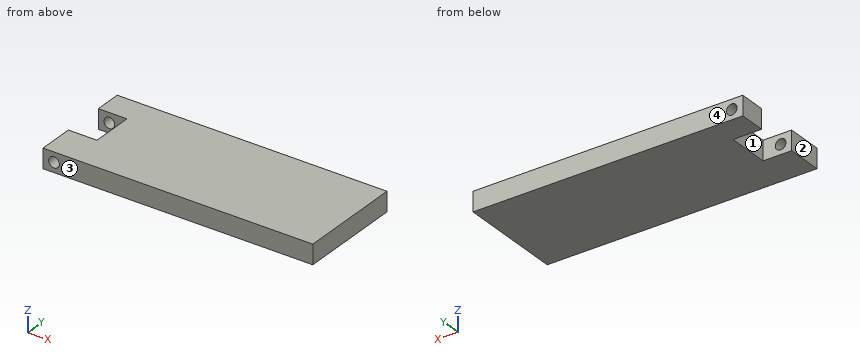
from build123d import *

# Parameters (mm, degrees)
F0_W     = 87.707184
F0_H     = 34.12497
F1_DEPTH = 6.35
F2_W     = 9.312924
F2_H     = 13.797991
F3_DEPTH = 6.35
F4_R     = 1.73945
F5_DEPTH = 34.12497


with BuildPart() as f1:
    # F0 (on Top) → F1 (new body)
    with BuildSketch(Plane.XY):
        with Locations((43.853592, 17.062485)):
            Rectangle(F0_W, F0_H)
    extrude(amount=F1_DEPTH)

    # F2 (on face) → F3 (cut, through all)
    with BuildSketch(Plane.XY.offset(6.35)):
        with Locations((4.656462, 18.549588)):
            Rectangle(F2_W, F2_H)
    extrude(amount=-F3_DEPTH, mode=Mode.SUBTRACT)

    # F4 (on face) → F5 (cut, through all)
    with BuildSketch(Plane(origin=(0, 34.12497, 0), x_dir=(-1, 0, 0), z_dir=(0, 1, 0))):
        with Locations((-3.584127, 3.175)):
            Circle(F4_R)
    extrude(amount=-F5_DEPTH, mode=Mode.SUBTRACT)


solid = f1.part
Work out the finished part from the listing and answer in its coordinate system (mm). Face numbers are marked on the shaded views. Coordinates: 2 decimals unless noted, no trailing zeros. Write each loop counter-clockwise with the first axis right and the second up, starting at its lowest first coordinate (ties: lowest second). Pieces come first, ordered by that corner, then holes. Notation, with made-up numbers: M 49,69.5 L 69,69.5 A20 ccw 69,92.5 Z; hole C 33,40.25 d4. An arc over 180 degrees is marked long. Answer as CSV lines item,"result". Start each with the question number.
Item 1: Determine the mould class of the marked faces 1, 2, 3 and 4 for opening direction Y: released by +Y, released by -Y, zero draft, split by the parting line, or undercut.
Item 2: Consider L1, parallel to X at y = 26.5, z = 3; L2, parallel to X at y = 14, z = 5; L3, parallel to X at y = 5, z = 4.25. Determine where each line is inside the solid, lowest interval first.
Item 3: Flat-ended cylindrical pins translate along their axes: P1, Ø1, axis at y = 23.5, z = 1, coming from the -X side; P2, Ø1.9, axis at x = 4.5, z = 2.5, coming from the +Y side. Find the tip coordinate at first contact, or state that the pin passes through.
Item 4: Section A-A on y = 31.5 is taken. Write down the section's boundary in (x, z) (3 decimals).
Item 5: Section B-B on y = 24.5 is taken. Write down the section's boundary in (x, z), and give its area (3 significant figures).
Checks:
1,face 1,"undercut"
1,face 2,"zero draft"
1,face 3,"released by -Y"
1,face 4,"released by +Y"
2,L1,"x = 0 to 1.85, 5.31 to 87.71"
2,L2,"x = 9.31 to 87.71"
2,L3,"x = 0 to 2.22, 4.95 to 87.71"
3,P1,"stops at x = 9.31"
3,P2,"stops at y = 34.12"
4,outline,"M 0,0 L 87.707,0 L 87.707,6.35 L 0,6.35 Z; hole C 3.584,3.175 d3.479"
5,outline,"M 9.31,0 L 87.71,0 L 87.71,6.35 L 9.31,6.35 Z"
5,area,"498 mm²"
